Here's the drawing with two shaded views (mm, measured from the low corner). I have some questions. A direction names the side the tool comes from. Round coordinates to 2 decimals unless told otherwise and drop trailing zeros. Order: outer loops, then holes, each group sorted by start corner. A loop starts at its lowest first (then second) coordinate and runs counter-clockwise, first axis right, second up.
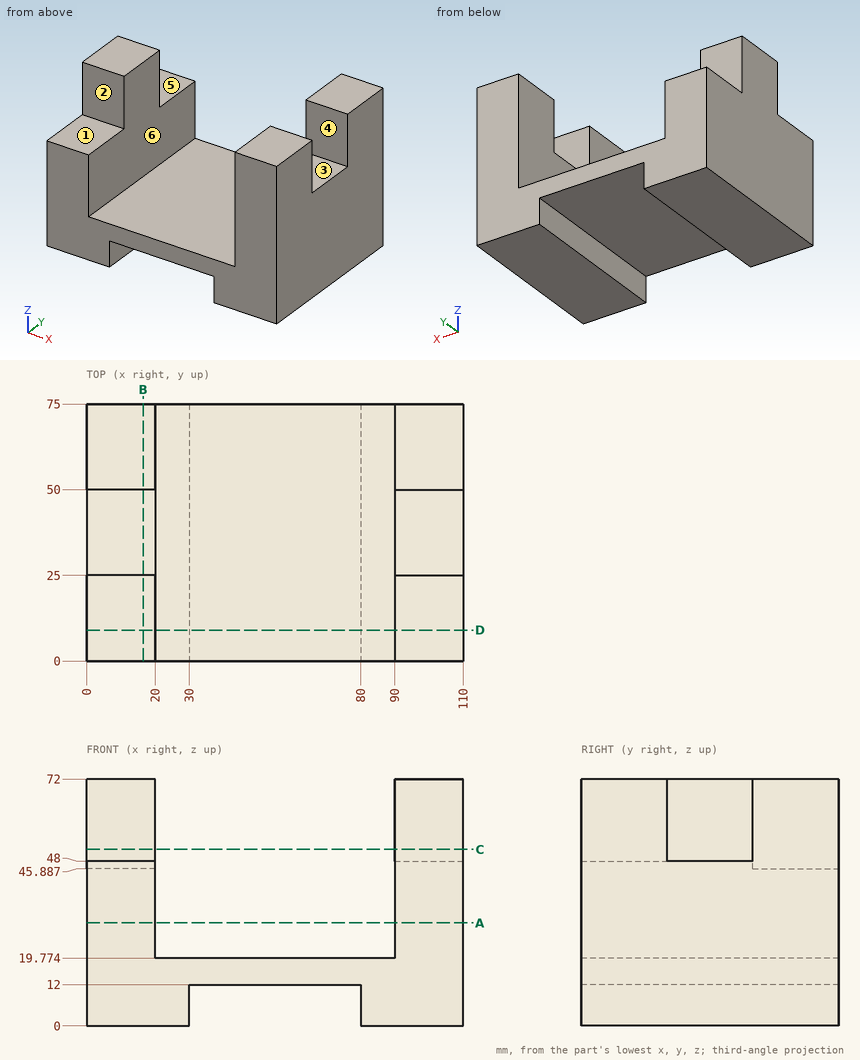
1. On a 3-axis mill with a long thin cutter (end or side, diameter ignored), from which of +Z, -Z, +X, -X, +Y, -Y can I reach the whole of each face in a straight line? I mean the marked faces 4, 5 and 6. Say none if no direction works.
Evaluation:
face 4: +Z, +X
face 5: +Z, -X, +Y
face 6: +Z, +Y, -Y
2. I'm going to push flat-ended pins straight in: P1, Ø10, axis at x = 5.5, z = 61.5, coming from the +Y side; P2, Ø22, axis at x = 14.5, y = 62, coming from the +Z side; P3, Ø3, axis at x = 32, y = 64.5, coming from the -Z side; P4, Ø1.5, axis at x = 49.5, z = 10, coming from the +Y side. Where does each tip first touch, or does it pass through?
Evaluation:
P1: stops at y = 50
P2: stops at z = 45.89
P3: stops at z = 12
P4: passes through
3. If we section it at D-D, the plane y = 9: Write out the boundary of the cut face in (x, z).
Evaluation:
outline: (0, 0) - (30, 0) - (30, 12) - (80, 12) - (80, 0) - (110, 0) - (110, 72) - (90, 72) - (90, 19.77) - (20, 19.77) - (20, 48) - (0, 48) - close
4. I need wall thicknesses on probe 1 along X at (y, z) = (20, 24); probe 2 along X at (y, z) = (18, 11); probe 3 along Y at (x, z) = (104, 59). Which ranges of each line are inside material? Lowest first, please.
Evaluation:
probe 1: x = 0 to 20, 90 to 110
probe 2: x = 0 to 30, 80 to 110
probe 3: y = 0 to 25, 50 to 75
5. If we mould it in two halves opening along Y, with no side actions, what happens to the marked faces 1, 2 and 3? For each: released by +Y, released by -Y, zero draft, split by the parting line, or undercut.
Evaluation:
face 1: zero draft
face 2: released by -Y
face 3: undercut
6. If we section it at C-C, the plane z = 51.5: Write out the boundary of the cut face in (x, y).
Evaluation:
outline: (0, 25) - (20, 25) - (20, 50) - (0, 50) - close; (90, 0) - (110, 0) - (110, 25) - (90, 25) - close; (90, 50) - (110, 50) - (110, 75) - (90, 75) - close
7. If we section it at B-B, the plane x = 16.5: Write out the boundary of the cut face in (y, z).
Evaluation:
outline: (0, 0) - (75, 0) - (75, 45.89) - (50, 45.89) - (50, 72) - (25, 72) - (25, 48) - (0, 48) - close
8. If we section it at A-A, the plane z = 30: Write out the boundary of the cut face in (x, y), and give its area (3 significant figures).
Evaluation:
outline: (0, 0) - (20, 0) - (20, 75) - (0, 75) - close; (90, 0) - (110, 0) - (110, 75) - (90, 75) - close
area: 3,000 mm2
